The listing builds one solid part. Answer for the finished solid, in the listing's coordinates (mm). Round coordinates to 2 decimals unless told otherwise and drop trailing zeros. Order: outer loops, then holes, each group sorted by start corner. A loop starts at its lowest first (then second) coordinate and runs counter-clockwise, first axis right, second up. Notation, with made-up numbers: (7, -36) - (56, -36) arc R5 ccw to (56, -27) - close; hole circle Ø8 at (36, 10.25). An arc over 180 degrees is marked (long way). Write item = value, one per line.
from build123d import *

# Parameters (mm, degrees)
ESQUISSE1_W             = 10
ESQUISSE1_H             = 10
BOSS_EXTRU_1_DEPTH      = 114.5
BOSS_EXTRU_1_DEPTH_BACK = 114.5
ESQUISSE2_R             = 1.6
ENL_V_MAT_EXTRU_1_DEPTH = 11


with BuildPart() as part:
    # Esquisse1 → Boss.-Extru.1 (new body, two sides)
    with BuildSketch(Plane.XY) as boss_extru_1_sk:
        Rectangle(ESQUISSE1_W, ESQUISSE1_H)
    extrude(amount=BOSS_EXTRU_1_DEPTH)
    extrude(boss_extru_1_sk.sketch, amount=-BOSS_EXTRU_1_DEPTH_BACK)

    # Esquisse2 → Enlèv. mat.-Extru.1 (cut, through all)
    with BuildSketch(Plane(origin=(0, 5, 0), x_dir=(1, 0, 0), z_dir=(0, 1, 0))):
        with Locations((0, 68)):
            Circle(ESQUISSE2_R)
        with Locations((0, -68)):
            Circle(ESQUISSE2_R)
    extrude(amount=-ENL_V_MAT_EXTRU_1_DEPTH, mode=Mode.SUBTRACT)


solid = part.part
Q1. A flat-ended cylindrical pin translates along its axis: P1, Ø1.9, axis at x = 0, z = 68, coming from the +Y side. Find the tip coordinate at first contact, or state that the pin passes through.
Model answer:
P1 = through
Q2. Find the intervals of material crossed by line 1 (Z direction, x = 0, y = 0.5); line 2 (X direction, y = -1, z = 68); line 3 (Z direction, x = -0.5, y = 2.5), in increasing order. Write a range as from..to.
Model answer:
line_1 = -114.5..-69.6, -66.4..66.4, 69.6..114.5
line_2 = -5..-1.6, 1.6..5
line_3 = -114.5..-69.52, -66.48..66.48, 69.52..114.5
Q3. Section A-A on x = 0 is taken. Determine the outline of the cut face in (y, z).
Model answer:
outline = (-5, -114.5) - (5, -114.5) - (5, -69.6) - (-5, -69.6) - close; (-5, -66.4) - (5, -66.4) - (5, 66.4) - (-5, 66.4) - close; (-5, 69.6) - (5, 69.6) - (5, 114.5) - (-5, 114.5) - close
